Geometry: final body of the model. Coordinates: model frame, mm. Face numbers are marked on the shaded views. Give positions to 0.01 mm unless a question says otherwise; leave off trailing zeros. Write each loop counter-clockwise with the first axis right and the second up, starting at its lowest first coordinate (ties: lowest second). Pieces come first, ordered by that corner, then holes. Notation, with made-up numbers: M 12,66 L 17,66 A12 cw 17,83 Z; hole C -8.75,72.25 d11. An arc over 180 degrees is marked long. Answer as a JSON object with one key per item and string values.
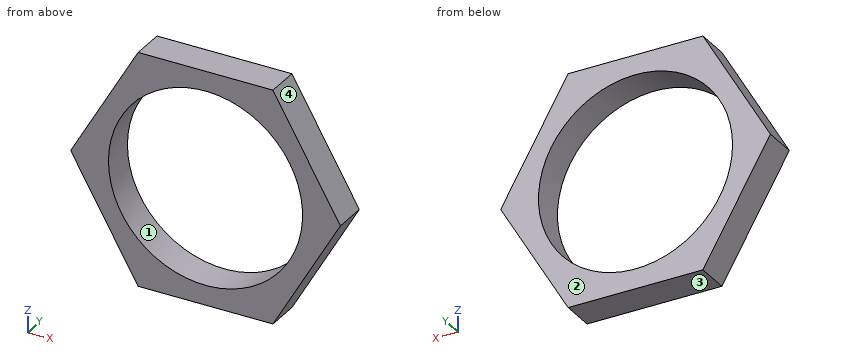
Autodesk Inventor part; units mm, degrees
ref_plane "YZ Plane" through (0, 0, 0) normal (1, 0, 0) x (0, 1, 0)
ref_plane "XZ Plane" through (0, 0, 0) normal (0, 1, 0) x (-1, 0, 0)
ref_plane "XY Plane" through (0, 0, 0) normal (0, 0, 1) x (1, 0, 0)
sketch "Sketch1" plane through (0, 0, 0) normal (0, 1, 0) x (-1, 0, 0)
  line L0 (6.4158, 11.1125) -> (12.8316, 0)
  line L1 (12.8316, 0) -> (6.4158, -11.1125)
  line L2 (6.4158, -11.1125) -> (-6.4158, -11.1125)
  line L3 (-6.4158, -11.1125) -> (-12.8316, 0)
  line L4 (-12.8316, 0) -> (-6.4158, 11.1125)
  line L5 (-6.4158, 11.1125) -> (6.4158, 11.1125)
  circle A0 centre (0, 0) radius 9.2329
  point P0 (0, 11.1125)
  dimension "d0" = 11.1125
  dimension "d1" = 18.4658
extrude "Extrusion1" add sketch "Sketch1" along normal blind 3.175
thread "Thread1"
properties part number "KeyLockNut"
1) Line query: line 1 (Z direction, x = 0, y = 2.05); line 2 (X direction, y = 1, z = 7); line 3 (Z direction, x = -2.25, y = 2.2). Output: solid intervals per line, ascending. Write a range as from..to.
Geometry check:
{"line 1": "z = -11.11..-9.23, 9.23..11.11", "line 2": "x = -8.79..-6.02, 6.02..8.79", "line 3": "z = -11.11..-8.95, 8.95..11.11"}
2) Cut plane A-A on y = 2.1. Return loops of the section in (x, z).
Geometry check:
{"outline": "M -12.83,0 L -6.42,-11.11 L 6.42,-11.11 L 12.83,0 L 6.42,11.11 L -6.42,11.11 Z; hole C 0,0 d18.47"}
3) Contact query for a flat-ended pin moving along its axis: P1, Ø1, axis at y = 1, z = 8.5, coming from the -X side. Output: stop coordinate, or through.
Geometry check:
{"P1": "stops at x = -8.21"}
4) Cut plane C-C on z = -4. Return loops of the section in (x, y) (3 decimals), and give its area (3 significant figures).
Geometry check:
{"outline": "M -10.522,0 L -8.321,0 L -8.321,3.175 L -10.522,3.175 Z; M 8.321,0 L 10.522,0 L 10.522,3.175 L 8.321,3.175 Z", "area": "14.0 mm2"}
5) Pull-direction query (Z, two-part tool) for the marked faces 1, 2, 3 and 4; classes: pulls with the +Z half, pulls with the -Z half, needs draft (parallel to the pull), parting line crosses it, or undercut.
Geometry check:
{"face 1": "undercut", "face 2": "needs draft", "face 3": "pulls with the -Z half", "face 4": "pulls with the +Z half"}
6) Cut plane D-D on x = 10.5. Return loops of the section in (y, z) (3 decimals).
Geometry check:
{"outline": "M 0,-4.038 L 3.175,-4.038 L 3.175,4.038 L 0,4.038 Z"}
7) Cut plane B-B on x = 0. Return loops of the section in (y, z) (1 decimal).
Geometry check:
{"outline": "M 0,-11.1 L 3.2,-11.1 L 3.2,-9.2 L 0,-9.2 Z; M 0,9.2 L 3.2,9.2 L 3.2,11.1 L 0,11.1 Z"}
